Can you work these out from the model? Positions are in its coordinate system, mm. A direction names the side the tool comes from. Coordinates: 2 decimals unless noted, no trailing zeros. Order: outer loops, then holes, each group sorted by start corner. A loop starts at its lowest first (then second) coordinate and runs counter-clockwise, first axis right, second up. Notation, with made-up numbers: M 33,86 L 46,86 A16 ccw 46,96 Z; hole C 36,8.5 d2. An arc over 180 degrees is marked long. Answer as a JSON object with one key per item and string values.
from build123d import *

# Parameters (mm, degrees)
SKETCH2_R           = 4.3
BOSS_EXTRUDE2_DEPTH = 35
CUT_EXTRUDE2_DEPTH  = 18
SKETCH6_R           = 0.75
CUT_EXTRUDE3_DEPTH  = 10
SKETCH8_R           = 0.75
CUT_EXTRUDE5_DEPTH  = 5.3
SKETCH9_R           = 0.75
CUT_EXTRUDE6_DEPTH  = 10


with BuildPart() as part:
    # Sketch2 → Boss-Extrude2 (new body)
    with BuildSketch(Plane(origin=(0, 0, 0), x_dir=(1, 0, 0), z_dir=(0, 1, 0))):
        Circle(SKETCH2_R)
    extrude(amount=BOSS_EXTRUDE2_DEPTH)

    # Sketch4 → Cut-Extrude2 (cut)
    with BuildSketch(Plane(origin=(0, 35, 0), x_dir=(1, 0, 0), z_dir=(0, 1, 0))):
        with BuildLine():
            Line((0, 2.15), (-3.723909236, 2.15))
            ThreePointArc((-3.723909236, 2.15), (0, 4.3), (3.723909236, 2.15))
            Line((3.723909236, 2.15), (0, 2.15))
        make_face()
        with BuildLine():
            Line((0, -2.15), (-3.723909236, -2.15))
            ThreePointArc((-3.723909236, -2.15), (0, -4.3), (3.723909236, -2.15))
            Line((3.723909236, -2.15), (0, -2.15))
        make_face()
    extrude(amount=-CUT_EXTRUDE2_DEPTH, mode=Mode.SUBTRACT)

    # Sketch6 → Cut-Extrude3 (cut)
    with BuildSketch(Plane.XY.offset(2.15)):
        with Locations((0, 19)):
            Circle(SKETCH6_R)
    extrude(amount=-CUT_EXTRUDE3_DEPTH, mode=Mode.SUBTRACT)

    # Sketch8 → Cut-Extrude5 (cut, through all)
    with BuildSketch(Plane(origin=(0, 0, 0), x_dir=(0, 0, -1), z_dir=(1, 0, 0))):
        with Locations((0, 1)):
            Circle(SKETCH8_R)
    extrude(amount=-CUT_EXTRUDE5_DEPTH, mode=Mode.SUBTRACT)

    # Sketch9 → Cut-Extrude6 (cut)
    with BuildSketch(Plane.XY.offset(2.15)):
        with Locations((0, 33.5)):
            Circle(SKETCH9_R)
    extrude(amount=-CUT_EXTRUDE6_DEPTH, mode=Mode.SUBTRACT)


solid = part.part
Item 1: I want a section at B-B, the plane z = 0. Write out the boundary of the cut face in (x, y), plus the area to 3 significant figures.
Answers follow:
{"outline": "M -4.3,0 L 4.3,0 L 4.3,35 L -4.3,35 L -4.3,1.75 L 0,1.75 L 0,0.25 L -4.3,0.25 Z; hole C 0,19 d1.5; hole C 0,33.5 d1.5", "area": "291 mm^2"}
Item 2: Please list where these lines run through material, in increasing order: line 1 (Y direction, x = 0, z = 1); line 2 (Y direction, x = -0.5, z = 1.5); line 3 (Z direction, x = -2.25, y = 19).
Answers follow:
{"line 1": "y = 0 to 18.25, 19.75 to 32.75, 34.25 to 35", "line 2": "y = 0 to 18.44, 19.56 to 32.94, 34.06 to 35", "line 3": "z = -2.15 to 2.15"}
Item 3: I want a section at A-A, the plane y = 19. Write out the boundary of the cut face in (x, z).
Answers follow:
{"outline": "M -3.72,-2.15 L -0.75,-2.15 L -0.75,2.15 L -3.72,2.15 A4.3 ccw Z; M 0.75,-2.15 L 3.72,-2.15 A4.3 ccw 3.72,2.15 L 0.75,2.15 Z"}
Item 4: If we mould it in two halves opening along Y, with no side actions, what happens to faces 4 (the cylindrical face through (-2.12, 0.268, 0.163)), 5 (the flat face through (0, 26, -2.15)), 6 (the flat face through (0, 17, -3)), 7 (the cylindrical face through (0.403, 34.132, 0.03))? For each: pulls with the +Y half, pulls with the -Y half, needs draft (parallel to the pull), parting line crosses it, or undercut.
Answers follow:
{"face 4": "undercut", "face 5": "needs draft", "face 6": "pulls with the +Y half", "face 7": "undercut"}
Item 5: I want a section at D-D, the plane z = -1.5. Write out the boundary of the cut face in (x, y), plus the area to 3 significant figures.
Answers follow:
{"outline": "M -4.03,0 L 4.03,0 L 4.03,35 L -4.03,35 Z; hole C 0,19 d1.5; hole C 0,33.5 d1.5", "area": "279 mm^2"}
Item 6: Which directions (+Z, -Z, +X, -X, +Y, -Y) give clear straight access to the entire face, cutting with the end or side of a thin tool? Please do faces 1 (the flat face through (0, 1, 0)), 2 (the flat face through (0, 17, 3)), 3 (the cylindrical face through (3.97, 13.37, 1.65)).
Answers follow:
{"face 1": "-X", "face 2": "+Z, +X, -X, +Y", "face 3": "+Y, -Y"}
Item 7: I'm going to push flat-ended pins straight in: pin 1 (4 mm diameter, centred on x = -1.5, z = 2, fed in from -Y); pin 2 (0.6 mm diameter, centred on x = 0, z = 4, fed in from +Y); pin 3 (3.5 mm diameter, centred on x = 0, y = 30, fed in from +Z); pin 4 (1.5 mm diameter, centred on y = 29.5, z = 2, fed in from +X). Where does each tip first touch, or does it pass through?
Answers follow:
{"pin 1": "stops at y = 0", "pin 2": "stops at y = 17", "pin 3": "stops at z = 2.15", "pin 4": "stops at x = 4.11"}
Item 8: I want a section at C-C, the plane x = -1.5. Write out the boundary of the cut face in (y, z).
Answers follow:
{"outline": "M 0,-4.03 L 17,-4.03 L 17,-2.15 L 35,-2.15 L 35,2.15 L 17,2.15 L 17,4.03 L 0,4.03 Z; hole C 1,0 d1.5"}
